Here's the drawing with two shaded views (mm, measured from the low corner). I have some questions. A direction names the side the tool comes from. Round coordinates to 2 decimals unless told otherwise and drop trailing zeros. Loops run counter-clockwise (first coordinate to the right, second up) from the corner with the lowest first, then second, coordinate; pieces in that order, holes last.
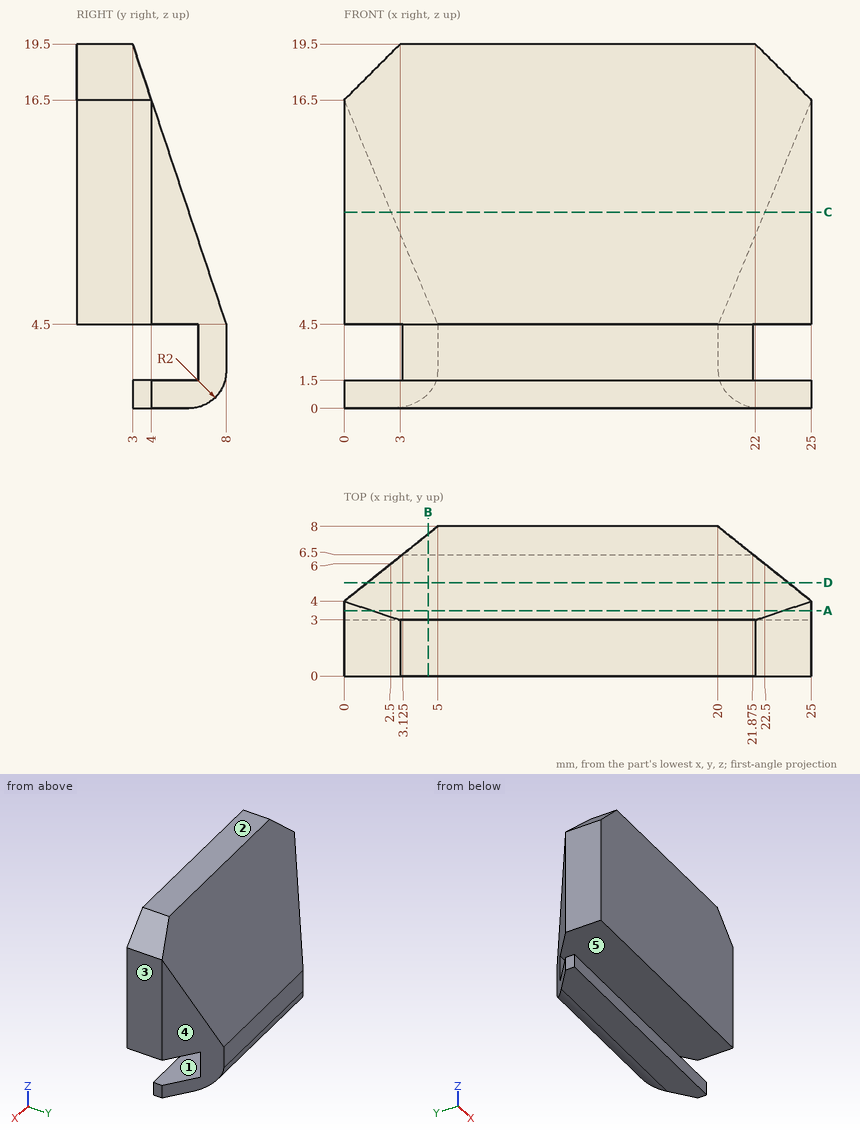
(1) If we section it at A-A, the plane y = 3.5: List the corners of the cut face in (x, z) for me, then the cut area to 3 significant figures.
Worked answers:
outline: (0, 0) - (25, 0) - (25, 1.5) - (0, 1.5) - close; (0, 4.5) - (25, 4.5) - (25, 16.5) - (23.5, 18) - (1.5, 18) - (0, 16.5) - close
area: 373 mm2
(2) For the marked faces 4 and 5, which set-ups out of +Z, -Z, +X, -X, +Y, -Y let a thin tool reach every point of the face, with its end or its side?
Worked answers:
face 4: +Z, -Z, +X, +Y
face 5: +X, -X, -Y
(3) If we section it at D-D, the plane y = 5: List the corners of the cut face in (x, z) for me, then the cut area to 3 significant figures.
Worked answers:
outline: (1.25, 0) - (23.75, 0) - (23.75, 1.5) - (1.25, 1.5) - close; (1.25, 4.5) - (23.75, 4.5) - (23.75, 13.5) - (1.25, 13.5) - close
area: 236 mm2
(4) If we section it at B-B, the plane x = 4.5: List the corners of the cut face in (y, z) for me.
Worked answers:
outline: (0, 4.5) - (6.5, 4.5) - (6.5, 1.5) - (3, 1.5) - (3, 0) - (6, 0) arc R2 ccw to (7.6, 0.8) - (7.6, 5.7) - (3, 19.5) - (0, 19.5) - close
(5) If we mould it in two halves opening along Z, with no side actions, what happens to the marked faces 1, 2 and 3? For each: released by +Z, released by -Z, zero draft, split by the parting line, or undercut.
Worked answers:
face 1: undercut
face 2: released by +Z
face 3: zero draft
(6) If I drill on line 1 (Y direction, x = 20, z = 16.5); line 2 (Y direction, x = 16.75, z = 10.5); line 3 (Z direction, x = 21.25, y = 2), over which ranges is the centre line in solid material (lowest first)?
Worked answers:
line 1: y = 0 to 4
line 2: y = 0 to 6
line 3: z = 4.5 to 19.5
(7) Will these pins go through, and if not, where does the flat tip stop? P1, Ø8, axis at x = 18.5, z = 14, coming from the +Y side; P2, Ø0.8, axis at x = 16, z = 0.5, coming from the -Y side; P3, Ø0.9, axis at x = 10, z = 2.5, coming from the -Y side.
Worked answers:
P1: stops at y = 6.17
P2: stops at y = 3
P3: stops at y = 6.5
(8) If we section it at C-C, the plane z = 10.5: List the corners of the cut face in (x, y) for me, then the cut area to 3 significant figures.
Worked answers:
outline: (0, 0) - (25, 0) - (25, 4) - (22.5, 6) - (2.5, 6) - (0, 4) - close
area: 145 mm2
